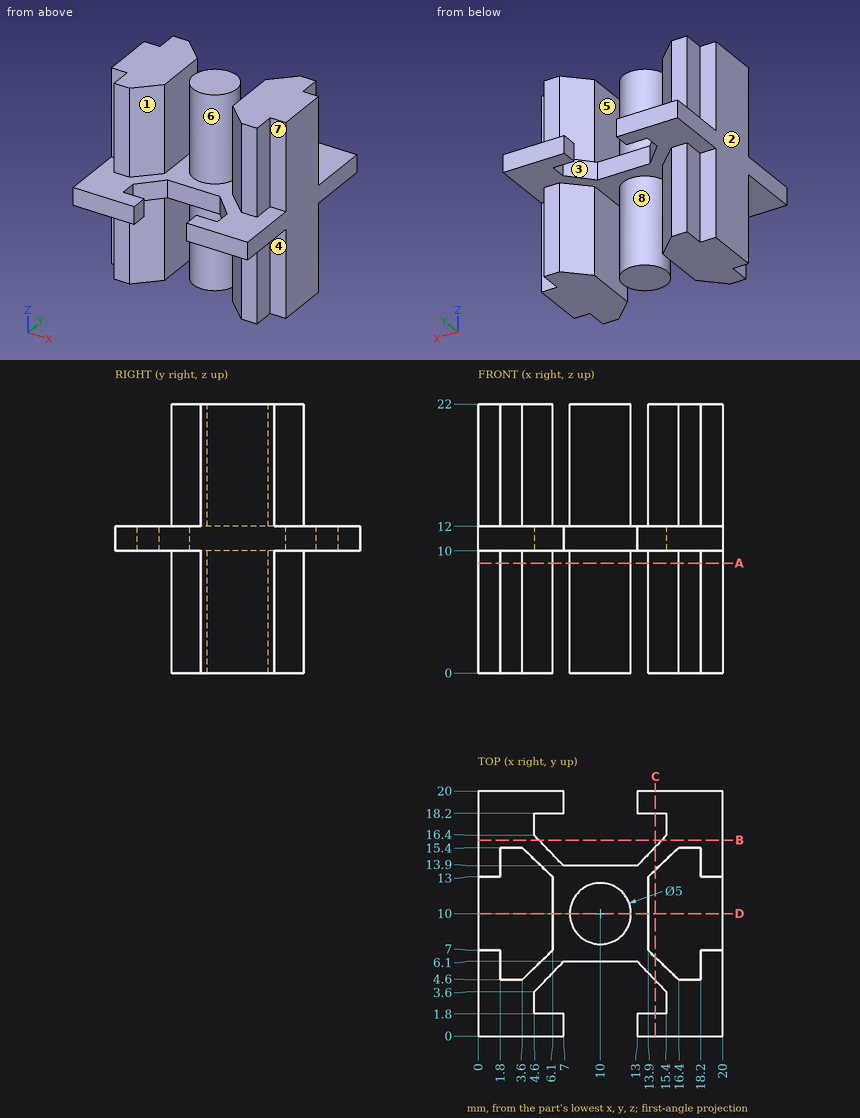
Could you check a few things on this drawing? It's one solid part, dimensions in mm from its lowest x, y, z. A direction names the side the tool comes from. Coordinates: 2 decimals unless noted, no trailing zeros. Write each loop counter-clockwise with the first axis right and the second up, starting at its lowest first coordinate (ties: lowest second). Pieces come first, ordered by that corner, then holes. Notation, with made-up numbers: (-15.75, -34) - (32.25, -34) arc R29 ccw to (32.25, -2) - close; hole circle Ø10 at (71, -7.5). An arc over 180 degrees is marked (long way). Return JSON: item names as keys, results as strings. Group by question number.
Item 1: We'd pull the mould along X, two halves only. Please class the marked faces 1, 2, 3 and 4: pulls with the +X half, pulls with the -X half, needs draft (parallel to the pull), parting line crosses it, or undercut.
Item 2: If we section it at A-A (z = 9): Write out the boundary of the cut face in (x, y), then the cut area to 3 significant figures.
Item 3: Which directions (+Z, -Z, +X, -X, +Y, -Y) give clear straight access to the entire face, cutting with the end or side of a thin tool? Please do the marked faces 5, 6, 7 and 8.
Item 4: If we section it at D-D (y = 10): Write out the boundary of the cut face in (x, z), then the cut area to 3 significant figures.
Item 5: If we section it at C-C (x = 14.5): Write out the boundary of the cut face in (y, z), then the cut area to 3 significant figures.
Item 6: If we section it at B-B (y = 16): Write out the boundary of the cut face in (x, z).
Item 7: Please list where these lines run through material, in increasing order: probe 1 along X at (y, z) = (12.25, 8); probe 2 along X at (y, z) = (8, 9.5); probe 3 along Y at (x, z) = (17, 4).
Item 8: I'm going to push flat-ended pins straight in: pin 1 Ø1.5 at (x, z) = (14, 2.5) entering from +Y; pin 2 Ø1.4 at (x, z) = (1, 7) entering from -Y; pin 3 Ø2 at (y, z) = (3.5, 4) entering from +X; pin 4 Ø6 at (x, y) = (5, 17.5) entering from -Z. Where does each tip first touch, or does it pass through?
Return value:
{
 "1": {"face 1": "undercut", "face 2": "pulls with the -X half", "face 3": "undercut", "face 4": "needs draft"},
 "2": {"outline": "(0, 7) - (1.8, 7) - (1.8, 4.6) - (3.6, 4.6) - (6.1, 7) - (6.1, 13) - (3.6, 15.4) - (1.8, 15.4) - (1.8, 13) - (0, 13) - close; circle Ø5 at (10, 10); (13.9, 7) - (16.4, 4.6) - (18.2, 4.6) - (18.2, 7) - (20, 7) - (20, 13) - (18.2, 13) - (18.2, 15.4) - (16.4, 15.4) - (13.9, 13) - close", "area": "122 mm^2"},
 "3": {"face 5": "+Z, +Y, -Y", "face 6": "+Z", "face 7": "+Z, +X, -Y", "face 8": "-Z"},
 "4": {"outline": "(0, 0) - (6.1, 0) - (6.1, 10) - (7.5, 10) - (7.5, 0) - (12.5, 0) - (12.5, 10) - (13.9, 10) - (13.9, 0) - (20, 0) - (20, 22) - (13.9, 22) - (13.9, 12) - (12.5, 12) - (12.5, 22) - (7.5, 22) - (7.5, 12) - (6.1, 12) - (6.1, 22) - (0, 22) - close", "area": "384 mm^2"},
 "5": {"outline": "(0, 10) - (1.8, 10) - (1.8, 12) - (0, 12) - close; (4.54, 10) - (6.42, 10) - (6.42, 0) - (13.58, 0) - (13.58, 10) - (15.46, 10) - (15.46, 12) - (13.58, 12) - (13.58, 22) - (6.42, 22) - (6.42, 12) - (4.54, 12) - close; (18.2, 10) - (20, 10) - (20, 12) - (18.2, 12) - close", "area": "172 mm^2"},
 "6": {"outline": "(0, 10) - (4.98, 10) - (4.98, 12) - (0, 12) - close; (15.02, 10) - (20, 10) - (20, 12) - (15.02, 12) - close"},
 "7": {"probe 1": "x = 0 to 6.1, 8.91 to 11.09, 13.9 to 20", "probe 2": "x = 0 to 6.1, 8.5 to 11.5, 13.9 to 20", "probe 3": "y = 4.6 to 15.4"},
 "8": {"pin 1": "stops at y = 13.82", "pin 2": "stops at y = 7", "pin 3": "passes through", "pin 4": "stops at z = 0"}
}
